Check sheet for the modelled part. Datum: model origin and axes. Units: mm. A direction names the side the tool comes from. Round coordinates to 2 decimals unless told otherwise and drop trailing zeros. Order: outer loops, then holes, each group sorted by start corner. A loop starts at its lowest first (then second) coordinate and runs counter-clockwise, first axis right, second up. Notation, with made-up numbers: (75.5, 55.25) -> (107.5, 55.25) arc R17 ccw to (107.5, 84.25) -> close; hole circle Ø3 at (-17, 67.5). An arc over 180 degrees is marked (long way). Answer in a Markdown table with one row per item.
```python
from build123d import *

# Parameters (mm, degrees)
EXTRUDE_1_DEPTH     = 9
SKETCH_2_W          = 4.5
SKETCH_2_H          = 6.5
EXTRUDE_2_DEPTH     = 17
SKETCH_3_W          = 9
SKETCH_3_H          = 1.5
CUT_EXTRUDE_1_DEPTH = 48.657633177


with BuildPart() as part:
    # Эскиз1 → Бобышка-Вытянуть1 (new body)
    with BuildSketch(Plane.XY):
        Polygon((-12.5, 12), (-12.5, -15), (5, -15), (5, 2), (12.5, 2), (12.5, 12), (3.5, 12), (3.5, 15), (-6.5, 15), (-6.5, 12), align=None)
    extrude_1 = extrude(amount=EXTRUDE_1_DEPTH)

    # Эскиз2 → Бобышка-Вытянуть2 (add)
    with BuildSketch(Plane.XZ.offset(15)):
        Polygon((-8, 15.5), (-8, 9), (-1.5, 9), (-1.5, 24), (-8, 24), align=None)
        with Locations((-10.25, 12.25)):
            Rectangle(SKETCH_2_W, SKETCH_2_H)
    extrude_2 = extrude(amount=-EXTRUDE_2_DEPTH)

    # Зеркальное отражение1: Бобышка-Вытянуть1, Бобышка-Вытянуть2 across plane
    add(extrude_1.mirror(Plane(origin=(-12.5, 0, 9), x_dir=(0, 0, 1), z_dir=(-1, 0, 0))))
    add(extrude_2.mirror(Plane(origin=(-12.5, 0, 9), x_dir=(0, 0, 1), z_dir=(-1, 0, 0))))

    # Эскиз3 → Вырез-Вытянуть1 (cut, through all)
    with BuildSketch(Plane(origin=(0, 2, 0), x_dir=(1, 0, 0), z_dir=(0, 1, 0))):
        with Locations((-12.5, -14.75)):
            Rectangle(SKETCH_3_W, SKETCH_3_H)
    extrude(amount=-CUT_EXTRUDE_1_DEPTH, mode=Mode.SUBTRACT)


solid = part.part
```
(1) Depth check by flat-ended pin: pin 1 Ø4.5 at (x, z) = (-14, 14) entering from +Y; pin 2 Ø11 at (y, z) = (-10.5, 21.5) entering from -X; pin 3 Ø7 at (y, z) = (-2.5, 4) entering from -X. Enter the tip coordinate at first touch or a pass-through.
Solutions:
| item | result |
|---|---|
| pin 1 | y = 2 |
| pin 2 | x = -23.5 |
| pin 3 | x = -30 |
(2) Section check D-D on z = 6. Record the boundary of the cut face in (x, y).
Solutions:
| item | result |
|---|---|
| outline | (-37.5, 2) -> (-30, 2) -> (-30, -15) -> (5, -15) -> (5, 2) -> (12.5, 2) -> (12.5, 12) -> (3.5, 12) -> (3.5, 15) -> (-6.5, 15) -> (-6.5, 12) -> (-18.5, 12) -> (-18.5, 15) -> (-28.5, 15) -> (-28.5, 12) -> (-37.5, 12) -> close |
(3) Section check B-B on y = 12.75. Record the boundary of the cut face in (x, z).
Solutions:
| item | result |
|---|---|
| outline | (-28.5, 0) -> (-18.5, 0) -> (-18.5, 9) -> (-28.5, 9) -> close; (-6.5, 0) -> (3.5, 0) -> (3.5, 9) -> (-6.5, 9) -> close |
(4) Section check C-C on y = -5.75. Record the boundary of the cut face in (x, z).
Solutions:
| item | result |
|---|---|
| outline | (-30, 0) -> (5, 0) -> (5, 9) -> (-1.5, 9) -> (-1.5, 24) -> (-8, 24) -> (-8, 14) -> (-17, 14) -> (-17, 24) -> (-23.5, 24) -> (-23.5, 9) -> (-30, 9) -> close |
(5) Draft check along X on faces 4 (the flat face through (-17, -7, 19)), 5 (the flat face through (-6.5, 14, 4)), 6 (the flat face through (-28.5, 13, 4)), 7 (the flat face through (-20, -7, 24)). Enter one of: pulls with the +X half, pulls with the -X half, needs draft (parallel to the pull), parting line crosses it, or undercut.
Solutions:
| item | result |
|---|---|
| face 4 | undercut |
| face 5 | undercut |
| face 6 | pulls with the -X half |
| face 7 | needs draft |
(6) Tool access check on faces 1 (the flat face through (-13, -6, 14)), 2 (the flat face through (-30, -7, 4)), 3 (the flat face through (-18.5, 14, 4)). Record the directions out of +Z, -Z, +X, -X, +Y, -Y that give a thin tool (end or side, any length) a straight path to the whole face; none if there is none.
Solutions:
| item | result |
|---|---|
| face 1 | +Z, +Y, -Y |
| face 2 | +Z, -Z, -X, -Y |
| face 3 | +Z, -Z, +Y |
(7) Scan lines: probe 1 along X at (y, z) = (-7, 16.5); probe 2 along X at (y, z) = (-6.25, 11.75); probe 3 along Y at (x, z) = (-32.5, 6.5). Record each from-to range of solid material in increasing order. Write a range as from..to.
Solutions:
| item | result |
|---|---|
| probe 1 | -23.5..-17, -8..-1.5 |
| probe 2 | -23.5..-1.5 |
| probe 3 | 2..12 |
(8) Section check A-A on z = 15.75. Record the boundary of the cut face in (x, y).
Solutions:
| item | result |
|---|---|
| outline | (-23.5, -15) -> (-17, -15) -> (-17, 2) -> (-23.5, 2) -> close; (-8, -15) -> (-1.5, -15) -> (-1.5, 2) -> (-8, 2) -> close |
